Can you work these out from the drawing? Everything is in mm from the part's minimum corner. Give positions to 0.01 mm unless a question says otherwise; leave off trailing zeros. Write each loop counter-clockwise with the first axis right and the second up, starting at its lowest first coordinate (ties: lowest second). Pieces come first, ordered by that corner, then holes. Notation, with made-up numbers: (34, 17.5) - (82, 17.5) arc R32 ccw to (82, 56.5) - close; hole circle Ø9 at (-0.75, -33.75). An arc over 180 degrees is marked (long way). Return JSON: item names as keys, results as strings. Group by question number.
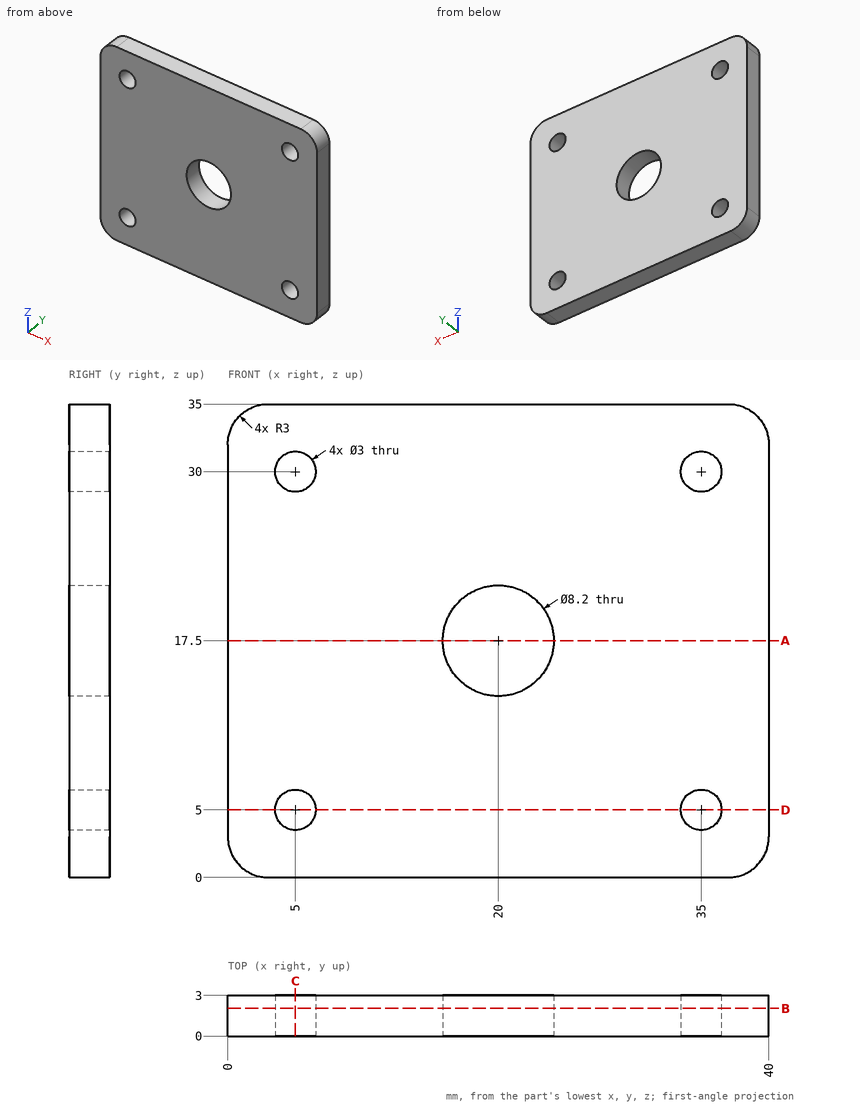
1) I need wall thicknesses on line 1 along X through (y, z) = (1.2, 5); line 2 along X through (y, z) = (1.3, 17.5); line 3 along X through (y, z) = (0.2, 16). Which ranges of each line are inside material? Lowest first, please.
2) Will these pins go through, and if not, where does the flat tip stop? pin 1 Ø2.5 at (x, z) = (35, 30) entering from -Y; pin 2 Ø6 at (x, z) = (27, 27.5) entering from -Y.
3) Imagine slicing it at D-D, the plane z = 5. Write out the boundary of the cut face in (x, y).
4) Imagine slicing it at C-C, the plane x = 5. Write out the boundary of the cut face in (y, z), and give its area (3 significant figures).
5) Imagine slicing it at A-A, the plane z = 17.5. Write out the boundary of the cut face in (x, y), and give its area (3 significant figures).
6) Imagine slicing it at B-B, the plane y = 2.05. Write out the boundary of the cut face in (x, z), and give its area (3 significant figures).
Resolved:
{
 "1": {"line 1": "0 to 3.5, 6.5 to 33.5, 36.5 to 40", "line 2": "0 to 15.9, 24.1 to 40", "line 3": "0 to 16.18, 23.82 to 40"},
 "2": {"pin 1": "through", "pin 2": "y = 0"},
 "3": {"outline": "(0, 0) - (3.5, 0) - (3.5, 3) - (0, 3) - close; (6.5, 0) - (33.5, 0) - (33.5, 3) - (6.5, 3) - close; (36.5, 0) - (40, 0) - (40, 3) - (36.5, 3) - close"},
 "4": {"outline": "(0, 0) - (3, 0) - (3, 3.5) - (0, 3.5) - close; (0, 6.5) - (3, 6.5) - (3, 28.5) - (0, 28.5) - close; (0, 31.5) - (3, 31.5) - (3, 35) - (0, 35) - close", "area": "87.0 mm^2"},
 "5": {"outline": "(0, 0) - (15.9, 0) - (15.9, 3) - (0, 3) - close; (24.1, 0) - (40, 0) - (40, 3) - (24.1, 3) - close", "area": "95.4 mm^2"},
 "6": {"outline": "(0, 3) arc R3 ccw to (3, 0) - (37, 0) arc R3 ccw to (40, 3) - (40, 32) arc R3 ccw to (37, 35) - (3, 35) arc R3 ccw to (0, 32) - close; hole circle Ø3 at (5, 5); hole circle Ø3 at (5, 30); hole circle Ø8.2 at (20, 17.5); hole circle Ø3 at (35, 5); hole circle Ø3 at (35, 30)", "area": "1,310 mm^2"}
}
